CAD build for the part. Positions are in the model's coordinates, mm. A direction names the side the tool comes from. Round coordinates to 2 decimals unless told otherwise and drop trailing zeros. Order: outer loops, then holes, each group sorted by start corner. A loop starts at its lowest first (then second) coordinate and runs counter-clockwise, first axis right, second up. Notation, with made-up numbers: (-9, -34.75) - (7, -34.75) arc R21 ccw to (7, -10.75) - close; hole circle Ø7 at (-21.75, 8.25). An arc over 180 degrees is marked (long way). Use one line per item in the form item = value. Start each with the question number.
from build123d import *

# Parameters (mm, degrees)
SKETCH1_W           = 4
SKETCH1_H           = 5
SKETCH2_R           = 2.5
BOSS_EXTRUDE1_DEPTH = 68.8
CUT_EXTRUDE1_START  = -15
CUT_EXTRUDE1_DEPTH  = 15
BOSS_EXTRUDE2_START = 60
SKETCH4_R           = 2.5
BOSS_EXTRUDE2_DEPTH = 60
CUT_EXTRUDE2_DEPTH  = 15
CHAMFER1_SIZE       = 0.5


with BuildPart() as part:
    # Sketch1 → Revolve1 (revolve)
    with BuildSketch(Plane(origin=(0, 0, 0), x_dir=(-1, 0, 0), z_dir=(0, 0, -1)), mode=Mode.PRIVATE) as revolve1_sk:
        with Locations((-7, 2.5)):
            Rectangle(SKETCH1_W, SKETCH1_H)
    revolve(revolve1_sk.sketch.rotate(Axis((9, 0, 0), (-1, 0, 0)), 270), axis=Axis((9, 0, 0), (-1, 0, 0)))

    # Sketch2 → Boss-Extrude1 (add)
    with BuildSketch(Plane(origin=(9, 0, 0), x_dir=(0, 0, -1), z_dir=(1, 0, 0))):
        with Locations(Location((0, 0, 0), (0, 0, 180))):
            Circle(SKETCH2_R)
    extrude(amount=BOSS_EXTRUDE1_DEPTH)

    # Sketch3 → Cut-Extrude1 (cut)
    with BuildSketch(Plane(origin=(77.8, 0, 0), x_dir=(0, 0, -1), z_dir=(1, 0, 0)).offset(CUT_EXTRUDE1_START)):
        with BuildLine():
            Line((-1.5, 2), (1.5, 2))
            ThreePointArc((1.5, 2), (0, 2.5), (-1.5, 2))
        make_face()
    extrude(amount=CUT_EXTRUDE1_DEPTH, mode=Mode.SUBTRACT)

    # Sketch4 → Boss-Extrude2 (add)
    with BuildSketch(Plane.ZY.offset(-5).offset(BOSS_EXTRUDE2_START)):
        with Locations(Location((0, 0, 0), (0, 0, 53.130102354))):
            Circle(SKETCH4_R)
    extrude(amount=-BOSS_EXTRUDE2_DEPTH)

    # Sketch5 → Cut-Extrude2 (cut)
    with BuildSketch(Plane.ZY.offset(55)):
        with BuildLine():
            Line((-1.5, 2), (1.5, 2))
            ThreePointArc((1.5, 2), (0, 2.5), (-1.5, 2))
        make_face()
    extrude(amount=-CUT_EXTRUDE2_DEPTH, mode=Mode.SUBTRACT)

    # Chamfer1
    chamfer1_edges = [part.edges().sort_by_distance(p)[0] for p in [
        (-55, -2.5, 0),
        (77.8, -2.236067977, -1.118033989),
    ]]
    chamfer(chamfer1_edges, length=CHAMFER1_SIZE - 0.0001)  # a hair under: the kernel refuses the full size


solid = part.part
(1) Slice it at C-C (x = 35). Give the cut face in (y, z), and give its area (3 significant figures).
(2) Flat gauge pins, fed straight in: P1, Ø6, axis at x = -37, z = 1, coming from the +Y side; P2, Ø4, axis at x = -21.5, y = 1.5, coming from the +Z side; P3, Ø1.5, axis at x = -48, z = 0, coming from the +Y side. Where does each tip first touch, or does it go through?
(3) Which spindle directions (+Z, -Z, +X, -X, +Y, -Y) get a long thin tool onto all of the face, cutting with end or side? Do faces 1 (the flat face through (5, -2, -2)), 2 (the flat face through (-48, 2, 0)), 3 (the flat face through (9, -2, -2)), 4 (the flat face through (77.8, 0, 0)), 5 (the flat face through (70, 2, 0)). Say none if no direction does.
(4) Slice it at B-B (x = -46). Give the cut face in (y, z), and give its area (3 significant figures).
(5) Slice it at A-A (y = 0). Give the cut face in (x, z).
(6) Wall check: line 1 (X direction, y = -1.5, z = -2.5); line 2 (Y direction, x = -5, z = 0.25); line 3 (Y direction, x = -43.5, z = -1.5). Give the ranges that are in metal, low to high. Write a range as [from, to].
Results list:
q1.outline = circle Ø5 at (0, 0)
q1.area = 19.6 mm²
q2.P1 = 2.5
q2.P2 = 2.5
q2.P3 = 2
q3.face_1 = -X
q3.face_2 = +Z, -Z, -X, +Y
q3.face_3 = +X
q3.face_4 = +Z, -Z, +X, +Y, -Y
q3.face_5 = +Z, -Z, +X, +Y
q4.outline = (2, -1.5) - (2, 1.5) arc R2.5 ccw (long way) to start
q4.area = 18.6 mm²
q5.outline = (-55, -2) - (-54.5, -2.5) - (5, -2.5) - (5, -5) - (9, -5) - (9, -2.5) - (77.3, -2.5) - (77.8, -2) - (77.8, 2) - (77.3, 2.5) - (9, 2.5) - (9, 5) - (5, 5) - (5, 2.5) - (-54.5, 2.5) - (-55, 2) - close
q6.line_1 = [5, 9]
q6.line_2 = [-2.49, 2.49]
q6.line_3 = [-2, 2]
